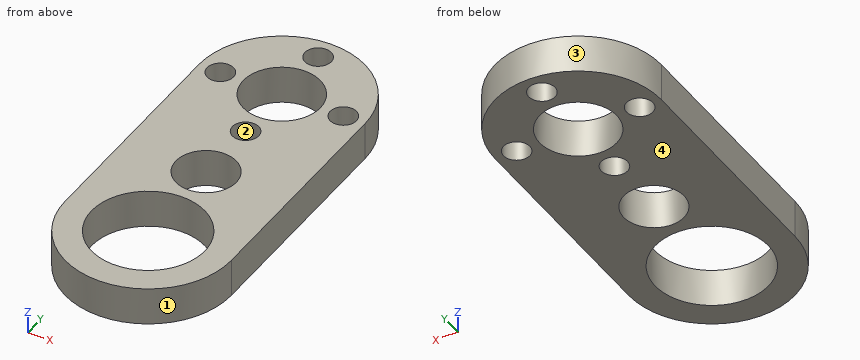
from build123d import *

# Parameters (mm, degrees)
ESBO_O1_R                = 11
ESBO_O1_R_2              = 5.105
RESSALTO_EXTRUS_O1_DEPTH = 5
ESBO_O2_R                = 1.75
CORTE_EXTRUS_O1_DEPTH    = 5
PADR_OCIRCULAR1_COUNT    = 4
ESBO_O3_R                = 7.5
ESBO_O3_R_2              = 4
RESSALTO_EXTRUS_O2_DEPTH = 5


with BuildPart() as part:
    # Esboço1 → Ressalto-extrusão1 (new body)
    with BuildSketch(Plane.XY):
        Circle(ESBO_O1_R)
        Circle(ESBO_O1_R_2, mode=Mode.SUBTRACT)
    extrude(amount=RESSALTO_EXTRUS_O1_DEPTH)

    # Esboço2 → Corte-extrusão1 (cut)
    with BuildSketch(Plane(origin=(0, 0, 0), x_dir=(-1, 0, 0), z_dir=(0, 0, -1))):
        with Locations((0, -8.14)):
            Circle(ESBO_O2_R)
    corte_extrus_o1 = extrude(amount=-CORTE_EXTRUS_O1_DEPTH, mode=Mode.SUBTRACT)

    # PadrãoCircular1: Corte-extrusão1 ×4 about axis
    padr_ocircular1_axis = Axis((0, 0, 0), (0, 0, 1))
    for i in range(1, PADR_OCIRCULAR1_COUNT):
        add(corte_extrus_o1.rotate(padr_ocircular1_axis, i * 360 / PADR_OCIRCULAR1_COUNT), mode=Mode.SUBTRACT)

    # Esboço3 → Ressalto-extrusão2 (add)
    with BuildSketch(Plane(origin=(0, 0, 0), x_dir=(-1, 0, 0), z_dir=(0, 0, -1))):
        with BuildLine():
            Line((-11, 0), (-11, -30))
            ThreePointArc((-11, -30), (0, -41), (11, -30))
            Line((11, -30), (11, 0))
            ThreePointArc((11, 0), (0, -11), (-11, 0))
        make_face()
        with Locations((0, -30)):
            Circle(ESBO_O3_R, mode=Mode.SUBTRACT)
        with Locations((0, -17)):
            Circle(ESBO_O3_R_2, mode=Mode.SUBTRACT)
    extrude(amount=-RESSALTO_EXTRUS_O2_DEPTH)


solid = part.part
Model file for the job. Use its own axes, mm. Face numbers are marked on the shaded views. Coordinates: 2 decimals unless noted, no trailing zeros. Order: outer loops, then holes, each group sorted by start corner. A loop starts at its lowest first (then second) coordinate and runs counter-clockwise, first axis right, second up. Notation, with made-up numbers: (89, 53.5) -> (125, 53.5) arc R21 cw to (125, 89.5) -> close; hole circle Ø3 at (74, 17). An arc over 180 degrees is marked (long way). Return JSON: item names as keys, results as strings. Group by question number.
Item 1: Saw through at D-D on x = 3. Write the cut outline in (y, z), then the cut area to 3 significant figures.
Item 2: Pull direction Y, two halves, no side cores. Call the marked faces 1, 2, 3 and 4: pulls with the +Y half, pulls with the -Y half, needs draft (parallel to the pull), parting line crosses it, or undercut.
Item 3: Flat gauge pins, fed straight in: P1, Ø3, axis at x = 0, y = -8.14, coming from the -Z side; P2, Ø3, axis at y = 5, z = 1, coming from the -X side; P3, Ø1, axis at x = -3, z = 2, coming from the -Y side. Where does each tip first touch, or does it go through?
Item 4: Wall check: line 1 along Y through (x, z) = (0, 1.45) (3 decimals); line 2 along X through (y, z) = (-24.5, 0.9); line 3 along Y through (x, z) = (1, 3.1). Give the ranges that are in metal, low to high. Write a range as [from, to].
Item 5: Saw through at C-C on z = 3.6. Write the cut outline in (x, y) (3 decimals), then the cut area to 3 significant figures.
Item 6: Saw through at B-B on x = 0. Write the cut outline in (y, z) (3 decimals), then the cut area to 4 significant figures.
Item 7: Saw through at A-A on y = -17. Write the cut outline in (x, z).
Values found:
{
 "1": {"outline": "(-40.58, 0) -> (-36.87, 0) -> (-36.87, 5) -> (-40.58, 5) -> close; (-23.13, 0) -> (-19.65, 0) -> (-19.65, 5) -> (-23.13, 5) -> close; (-14.35, 0) -> (-4.13, 0) -> (-4.13, 5) -> (-14.35, 5) -> close; (4.13, 0) -> (10.58, 0) -> (10.58, 5) -> (4.13, 5) -> close", "area": "119 mm2"},
 "2": {"face 1": "pulls with the -Y half", "face 2": "undercut", "face 3": "pulls with the +Y half", "face 4": "needs draft"},
 "3": {"P1": "passes through", "P2": "stops at x = -10.43", "P3": "stops at y = -40.71"},
 "4": {"line 1": "y = [-41, -37.5], [-22.5, -21], [-13, -9.89], [-6.39, -5.105], [5.105, 6.39], [9.89, 11]", "line 2": "x = [-11, -5.1], [5.1, 11]", "line 3": "y = [-40.95, -37.43], [-22.57, -20.87], [-13.13, -9.58], [-6.7, -5.01], [5.01, 6.7], [9.58, 10.95]"},
 "5": {"outline": "(-11, -30) arc R11 ccw to (11, -30) -> (11, 0) arc R11 ccw to (-11, 0) -> close; hole circle Ø3.5 at (-8.14, 0); hole circle Ø15 at (0, -30); hole circle Ø10.21 at (0, 0); hole circle Ø8 at (0, -17); hole circle Ø3.5 at (0, -8.14); hole circle Ø3.5 at (0, 8.14); hole circle Ø3.5 at (8.14, 0)", "area": "693 mm2"},
 "6": {"outline": "(-41, 0) -> (-37.5, 0) -> (-37.5, 5) -> (-41, 5) -> close; (-22.5, 0) -> (-21, 0) -> (-21, 5) -> (-22.5, 5) -> close; (-13, 0) -> (-9.89, 0) -> (-9.89, 5) -> (-13, 5) -> close; (-6.39, 0) -> (-5.105, 0) -> (-5.105, 5) -> (-6.39, 5) -> close; (5.105, 0) -> (6.39, 0) -> (6.39, 5) -> (5.105, 5) -> close; (9.89, 0) -> (11, 0) -> (11, 5) -> (9.89, 5) -> close", "area": "58.95 mm2"},
 "7": {"outline": "(-11, 0) -> (-4, 0) -> (-4, 5) -> (-11, 5) -> close; (4, 0) -> (11, 0) -> (11, 5) -> (4, 5) -> close"}
}
